```python
from build123d import *

# Parameters (mm, degrees)
SKETCH1_R               = 7.5
BOSS_EXTRUDE1_DEPTH     = 6
BOSS_EXTRUDE2_DEPTH     = 4
BOSS_EXTRUDE3_DEPTH     = 2
CUT_EXTRUDE1_DEPTH      = 29.893122019
CUT_EXTRUDE1_DEPTH_BACK = 29.893122019
SKETCH5_R               = 1.5
SKETCH5_R_2             = 3
FILLET1_R               = 10


with BuildPart() as part:
    # Sketch1 → Boss-Extrude1 (new body)
    with BuildSketch(Plane(origin=(0, 0, 0), x_dir=(1, 0, 0), z_dir=(0, 1, 0))):
        with Locations(Location((0, 0, 0), (0, 0, 270))):
            Circle(SKETCH1_R)
    extrude(amount=BOSS_EXTRUDE1_DEPTH)

    # Sketch2 → Boss-Extrude2 (add)
    with BuildSketch(Plane(origin=(0, 6, 0), x_dir=(1, 0, 0), z_dir=(0, 1, 0))):
        with BuildLine():
            Line((0, 3.25), (24, 3.25))
            ThreePointArc((24, 3.25), (27.25, 0), (24, -3.25))
            Line((24, -3.25), (0, -3.25))
            ThreePointArc((0, -3.25), (-3.25, 0), (0, 3.25))
        make_face()
    extrude(amount=-BOSS_EXTRUDE2_DEPTH)

    # Sketch4 → Boss-Extrude3 (add)
    with BuildSketch(Plane(origin=(0, 2, 0), x_dir=(-1, 0, 0), z_dir=(0, -1, 0))):
        with BuildLine():
            Line((-24, 2.8), (-20.1, 2.8))
            ThreePointArc((-20.1, 2.8), (-17.3, 0), (-20.1, -2.8))
            Line((-20.1, -2.8), (-24, -2.8))
            ThreePointArc((-24, -2.8), (-26.8, 0), (-24, 2.8))
        make_face()
    extrude(amount=BOSS_EXTRUDE3_DEPTH)

    # Sketch5 → Cut-Extrude1 (cut, two sides: drawn at the far end of the back side and taken through both)
    with BuildSketch(Plane.XZ.offset(-CUT_EXTRUDE1_DEPTH_BACK)):
        with Locations(Location((24, 0, 0), (0, 0, 270))):
            Circle(SKETCH5_R)
        with Locations(Location((20.1, 0, 0), (0, 0, 270))):
            Circle(SKETCH5_R)
        with Locations(Location((0, 0, 0), (0, 0, 270))):
            Circle(SKETCH5_R_2)
    extrude(amount=CUT_EXTRUDE1_DEPTH + CUT_EXTRUDE1_DEPTH_BACK, mode=Mode.SUBTRACT)

    # Fillet1
    fillet1_edges = [part.edges().sort_by_distance(p)[0] for p in [
        (6.759252917, 4, -3.25),
        (6.759252917, 4, 3.25),
    ]]
    fillet(fillet1_edges, radius=FILLET1_R)


solid = part.part
```
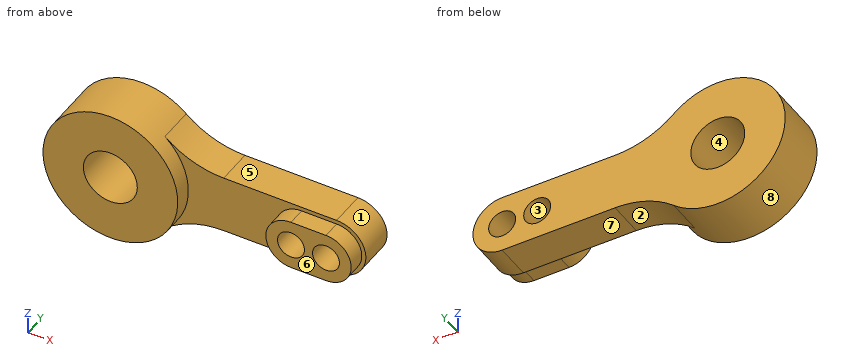
Input: part model. Units: mm. Frame: model coordinates. Face numbers are marked on the shaded views. A direction names the side the tool comes from. Give positions to 0.01 mm unless a question says otherwise; leave off trailing zeros. Order: outer loops, then holes, each group sorted by start corner. A loop starts at its lowest first (then second) coordinate and runs counter-clockwise, first axis right, second up. Notation, with made-up numbers: (89, 70) - (139, 70) arc R17 ccw to (139, 80) - close; hole circle Ø4 at (68.25, 27.25). An arc over 180 degrees is marked (long way). Put each result on its own line as item: value.
Item 1: Ray query, L1, parallel to X at y = 3.75, z = 0; L2, parallel to Z at x = 24, y = 1.3; L3, parallel to Y at x = 12, z = 1.25. Return the intervals inside material, ascending. Write a range as from..to.
Found:
L1: x = -7.5..-3, 3..18.6, 21.6..22.5, 25.5..27.25
L2: z = -2.8..-1.5, 1.5..2.8
L3: y = 2..6
Item 2: Section query A-A, the plane x = 0. Return loops of the section in (y, z).
Found:
outline: (0, -7.5) - (6, -7.5) - (6, -3) - (0, -3) - close; (0, 3) - (6, 3) - (6, 7.5) - (0, 7.5) - close
Item 3: Section query B-B, the plane z = 0. Return loops of the section in (x, y), then the cut area to 3 significant figures.
Found:
outline: (-7.5, 0) - (-3, 0) - (-3, 6) - (-7.5, 6) - close; (3, 0) - (7.5, 0) - (7.5, 2) - (17.3, 2) - (17.3, 0) - (18.6, 0) - (18.6, 6) - (3, 6) - close; (21.6, 0) - (22.5, 0) - (22.5, 6) - (21.6, 6) - close; (25.5, 0) - (26.8, 0) - (26.8, 2) - (27.25, 2) - (27.25, 6) - (25.5, 6) - close
area: 116 mm^2
Item 4: Section query D-D, the plane x = 18. Return loops of the section in (y, z), then the cut area to 3 significant figures.
Found:
outline: (0, -1.85) - (2, -1.85) - (2, -3.25) - (6, -3.25) - (6, 3.25) - (2, 3.25) - (2, 1.85) - (0, 1.85) - close
area: 33.4 mm^2
Item 5: Section query C-C, the plane y = 4.4. Return loops of the section in (x, z), then the cut area to 3 significant figures.
Found:
outline: (4.9, -5.68) arc R10 cw to (11.43, -3.25) - (24, -3.25) arc R3.25 ccw to (24, 3.25) - (11.43, 3.25) arc R10 cw to (4.9, 5.68) arc R7.5 ccw (long way) to start; hole circle Ø6 at (0, 0); hole circle Ø3 at (20.1, 0); hole circle Ø3 at (24, 0)
area: 265 mm^2
Item 6: Draft query along Z for the marked faces 1, 2, 3 and 4. Return one class per face: +Z half, -Z half, draft (parallel to the pull), parting line (faces both ways), or undercut.
Found:
face 1: parting line
face 2: -Z half
face 3: undercut
face 4: undercut
Item 7: Contact query for flat-ended pins moving along their axis: pin 1 (1.2 mm diameter, centred on x = 20, y = 3.5, fed in from -Z); pin 2 (3.5 mm diameter, centred on x = 17, z = 2.5, fed in from -Y). Output: stop coordinate, or through.
Found:
pin 1: stops at z = -3.25
pin 2: stops at y = 0
Item 8: Access query for the marked faces 5, 6, 7 and 8. Directions: +Z, -Z, +X, -X, +Y, -Y. A direction counts if a zero-diameter tool reaches every point of the face in a straight line with its end or side. Return the directions, or none.
Found:
face 5: +Z, +X, +Y, -Y
face 6: +Z, -Z, +X, -X, -Y
face 7: -Z, +X, +Y, -Y
face 8: -Y
